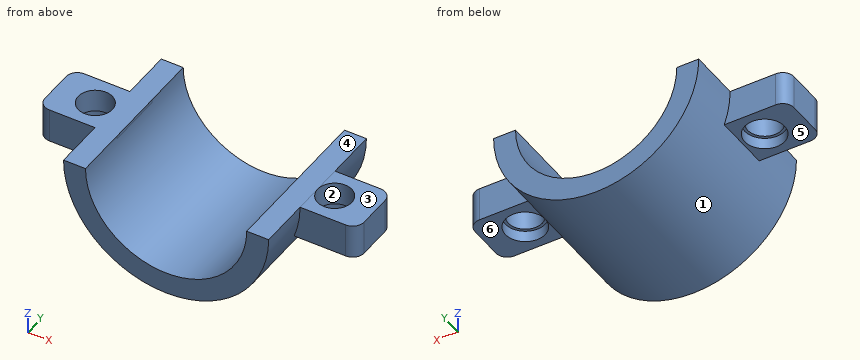
```python
from build123d import *

# Parameters (mm, degrees)
PAD037_DEPTH        = 13
PAD037_DEPTH_BACK   = 1
SKETCH058_W         = 1.93
SKETCH058_H         = 5
PAD038_DEPTH        = 3
SKETCH059_W         = 5
SKETCH059_H         = 3
PAD039_DEPTH        = 5
SKETCH060_W         = 5
SKETCH060_H         = 3
PAD040_DEPTH        = 5
HOLE005_D           = 3
HOLE005_DEPTH       = 3
HOLE005_CBORE_D     = 3.5
HOLE005_CBORE_DEPTH = 1
HOLE005_TIPS_R      = 1.5
FILLET010_R         = 1
FILLET011_R         = 1
FILLET012_R         = 1


with BuildPart() as part:
    # Sketch057 (on Face1 of CopyPad023) → Pad037 (new body, two sides)
    with BuildSketch(Plane(origin=(0, -35.363644, -2), x_dir=(1, 0, 0), z_dir=(0, -1, 0))) as pad037_sk:
        with BuildLine():
            ThreePointArc((-25.035308, -10.895555), (-17.960308, -17.970555), (-10.885308, -10.895554))
            Line((-10.885308, -10.895554), (-8.960308, -10.895554))
            ThreePointArc((-26.960308, -10.895555), (-17.960308, -19.895555), (-8.960308, -10.895554))
            Line((-26.960308, -10.895555), (-25.035308, -10.895555))
        make_face()
    extrude(amount=-PAD037_DEPTH)
    extrude(pad037_sk.sketch, amount=PAD037_DEPTH_BACK)

    # Sketch058 (on Face1 of Pad037) → Pad038 (join)
    with BuildSketch(Plane.XY.offset(-12.895555)):
        with Locations((-25.995308, -29.363644)):
            Rectangle(SKETCH058_W, SKETCH058_H)
        with Locations((-9.920308, -29.363644)):
            Rectangle(SKETCH058_W, SKETCH058_H)
    extrude(amount=-PAD038_DEPTH)

    # Sketch059 (on Face12 of Pad038) → Pad039 (join)
    with BuildSketch(Plane(origin=(-26.960308, 0, -2), x_dir=(0, -1, 0), z_dir=(-1, 0, 0))):
        with Locations((29.363644, -12.395555)):
            Rectangle(SKETCH059_W, SKETCH059_H)
    extrude(amount=PAD039_DEPTH)

    # Sketch060 (on Face13 of Pad039) → Pad040 (join)
    with BuildSketch(Plane(origin=(-8.955308, 0, -2), x_dir=(0, 1, 0), z_dir=(1, 0, 0))):
        with Locations((-29.363644, -12.395555)):
            Rectangle(SKETCH060_W, SKETCH060_H)
    extrude(amount=PAD040_DEPTH)

    # Hole005
    with Locations(Plane(origin=(0, 0, -15.895555), x_dir=(1, 0, 0), z_dir=(0, 0, -1))):
        with Locations((-7.455308, 29.363644), (-28.460308, 29.363644)):
            CounterBoreHole(HOLE005_D / 2, HOLE005_CBORE_D / 2, HOLE005_CBORE_DEPTH, depth=HOLE005_DEPTH)

    # Hole005 tips → Hole005 tip 1 section 0
    with BuildSketch(Plane(origin=(0, 0, -12.895555), x_dir=(1, 0, 0), z_dir=(0, 0, -1)), mode=Mode.PRIVATE) as hole005_tip_1_s0:
        with Locations((-7.455308, 29.363644)):
            Circle(HOLE005_TIPS_R)
    loft([hole005_tip_1_s0.sketch, Vertex(-7.455308, -29.363644, -11.994264)], mode=Mode.SUBTRACT)

    # Hole005 tips → Hole005 tip 2 section 0
    with BuildSketch(Plane(origin=(0, 0, -12.895555), x_dir=(1, 0, 0), z_dir=(0, 0, -1)), mode=Mode.PRIVATE) as hole005_tip_2_s0:
        with Locations((-28.460308, 29.363644)):
            Circle(HOLE005_TIPS_R)
    loft([hole005_tip_2_s0.sketch, Vertex(-28.460308, -29.363644, -11.994264)], mode=Mode.SUBTRACT)

    # Fillet010
    fillet010_edges = [part.edges().sort_by_distance(p)[0] for p in [
        (-31.960308, -31.863644, -14.395555),
    ]]
    fillet(fillet010_edges, radius=FILLET010_R)

    # Fillet011
    fillet011_edges = [part.edges().sort_by_distance(p)[0] for p in [
        (-31.960308, -26.863644, -14.395555),
    ]]
    fillet(fillet011_edges, radius=FILLET011_R)

    # Fillet012
    fillet012_edges = [part.edges().sort_by_distance(p)[0] for p in [
        (-3.955308, -26.863644, -14.395555),
        (-3.955308, -31.863644, -14.395555),
    ]]
    fillet(fillet012_edges, radius=FILLET012_R)


with BuildPart() as part_1:
    # Body007 placement: moved
    add(part.part.moved(Location((0.45, 32.66415, 1.7))))


solid = part_1.part
```
Input: part model. Units: mm. Frame: model coordinates. Face numbers are marked on the shaded views. A direction names the side the tool comes from. Give positions to 0.01 mm unless a question says otherwise; leave off trailing zeros. Order: outer loops, then holes, each group sorted by start corner. A loop starts at its lowest first (then second) coordinate and runs counter-clockwise, first axis right, second up.
1. Section D-D on z = -11.75. Return the cut outline in (x, y), and give its area (3 significant figures).
Derived:
outline: (-31.51, 1.8) arc R1 ccw to (-30.51, 0.8) - (-26.49, 0.8) - (-26.49, -3.7) - (-24.56, -3.7) - (-24.56, 10.3) - (-26.49, 10.3) - (-26.49, 5.8) - (-30.51, 5.8) arc R1 ccw to (-31.51, 4.8) - close; (-10.46, -3.7) - (-8.53, -3.7) - (-8.53, 0.8) - (-4.51, 0.8) arc R1 ccw to (-3.51, 1.8) - (-3.51, 4.8) arc R1 ccw to (-4.51, 5.8) - (-8.53, 5.8) - (-8.53, 10.3) - (-10.46, 10.3) - close; hole circle Ø3 at (-28.01, 3.3); hole circle Ø3 at (-7.01, 3.3)
area: 89.2 mm2
2. Mould query, pull axis X, two halves, no side actions, for the marked faces 1, 2 and 3. Classes: released by +X, released by -X, zero draft, split by the parting line, or undercut.
Derived:
face 1: split by the parting line
face 2: undercut
face 3: zero draft
3. Reachability of the marked faces 4, 5 and 6 from +Z, -Z, +X, -X, +Y, -Y: full face, straight path, thin tool, end or side. Return the list, or none.
Derived:
face 4: +Z, +X, -X, +Y, -Y
face 5: -Z, -X, +Y, -Y
face 6: -Z, +X, +Y, -Y
4. Pin query (flat end, axial travel): pin 1 (1 mm diameter, centred on x = -28, y = 3, fed in from -Z); pin 2 (5.5 mm diameter, centred on x = -29.5, y = 3.5, fed in from -Z); pin 3 (8 mm diameter, centred on x = -19.5, y = 2, fed in from +Z); pin 4 (1.5 mm diameter, centred on y = 2, z = -15.5, fed in from +X). Return the tip coordinate at first contact, or that it passes through.
Derived:
pin 1: passes through
pin 2: stops at z = -14.2
pin 3: stops at z = -14.96
pin 4: stops at x = -9.24
5. Section A-A on z = -15. Return the cut outline in (x, y).
Derived:
outline: (-25.67, -3.7) - (-23.48, -3.7) - (-23.48, 10.3) - (-25.67, 10.3) - close; (-11.55, -3.7) - (-9.35, -3.7) - (-9.35, 10.3) - (-11.55, 10.3) - close
6. Material intervals for L1, parallel to X at y = 2.25, z = -13; L2, parallel to X at y = 3.75, z = -16.25; L3, parallel to X at y = 4, z = -12.5, sorted ascending.
Derived:
L1: x = -31.51 to -29.08, -26.94 to -24.35, -10.67 to -8.08, -5.93 to -3.51
L2: x = -24.96 to -22.46, -12.56 to -10.06
L3: x = -31.51 to -29.34, -26.68 to -24.46, -10.56 to -8.33, -5.68 to -3.51
7. Section C-C on x = -28.25. Return the cut outline in (y, z), and give its area (3 significant figures).
Derived:
outline: (0.8, -14.2) - (1.57, -14.2) - (1.57, -13.2) - (1.82, -13.2) - (1.82, -11.2) - (0.8, -11.2) - close; (4.78, -13.2) - (5.03, -13.2) - (5.03, -14.2) - (5.8, -14.2) - (5.8, -11.2) - (4.78, -11.2) - close
area: 5.61 mm2
8. Section B-B on y = 4.5. Give the number of separate pieces and of enclosed holes in the cut face, and give its area (3 significant figures).
Derived:
separate pieces: 3
enclosed holes: 0
area: 67.3 mm2
